The listing builds one solid part. Answer for the finished solid, in the listing's coordinates (mm). A direction names the side the tool comes from. Give positions to 0.01 mm unless a question says otherwise; leave off trailing zeros. Order: outer loops, then holes, each group sorted by start corner. A loop starts at its lowest first (then second) coordinate and runs counter-clockwise, first axis right, second up. Notation, with made-up numbers: M 18,68.25 L 39,68.25 A32 ccw 39,103.25 Z; hole C 42,-18 d2. An arc over 180 degrees is marked long. Answer as a JSON object with one key per item and string values. Group by question number.
```python
from build123d import *

# Parameters (mm, degrees)
BOSS_EXTRUDE1_DEPTH = 1.5
BOSS_EXTRUDE2_DEPTH = 3.5
CUT_EXTRUDE1_DEPTH  = 4
FILLET1_R           = 1
FILLET4_R           = 1
SKETCH5_R           = 1.5
CUT_EXTRUDE3_DEPTH  = 12
SKETCH4_R           = 1
CUT_EXTRUDE5_DEPTH  = 20


with BuildPart() as part:
    # Sketch1 → Boss-Extrude1 (new body)
    with BuildSketch(Plane.XY):
        with BuildLine():
            Line((0, 0), (20, 0))
            Line((20, 0), (20, 16))
            Line((20, 16), (18, 16))
            ThreePointArc((18, 16), (0, 22.408858912), (-18, 16))
            Line((-18, 16), (-20, 16))
            Line((-20, 16), (-20, 0))
            Line((-20, 0), (0, 0))
        make_face()
    extrude(amount=BOSS_EXTRUDE1_DEPTH)

    # Sketch2 → Boss-Extrude2 (add)
    with BuildSketch(Plane.XY.offset(1.5)):
        with BuildLine():
            Line((6, 0), (6, 13))
            ThreePointArc((6, 13), (0, 19), (-6, 13))
            Line((-6, 13), (-6, 0))
            Line((-6, 0), (6, 0))
        make_face()
    extrude(amount=BOSS_EXTRUDE2_DEPTH)

    # Sketch3 → Cut-Extrude1 (cut)
    with BuildSketch(Plane(origin=(0, 0, 0), x_dir=(-1, 0, 0), z_dir=(0, 0, -1))):
        with BuildLine():
            Line((0, 0), (5, 0))
            Line((5, 0), (5, 12))
            ThreePointArc((5, 12), (0, 17), (-5, 12))
            Line((-5, 12), (-5, 0))
            Line((-5, 0), (0, 0))
        make_face()
    extrude(amount=-CUT_EXTRUDE1_DEPTH, mode=Mode.SUBTRACT)

    # Fillet1
    fillet1_edges = [part.edges().sort_by_distance(p)[0] for p in [
        (-6, 6.5, 5),
        (0, 19, 5),
        (0, 0, 5),
        (6, 6.5, 5),
    ]]
    fillet(fillet1_edges, radius=FILLET1_R - 0.0001)  # a hair under: the kernel refuses the full size

    # Fillet4
    fillet4_edges = [part.edges().sort_by_distance(p)[0] for p in [
        (20, 8, 1.5),
        (19, 16, 1.5),
        (0, 22.408858912, 1.5),
        (13, 0, 1.5),
        (-19, 16, 1.5),
        (-20, 8, 1.5),
        (-13, 0, 1.5),
    ]]
    fillet(fillet4_edges, radius=FILLET4_R)

    # Sketch5 → Cut-Extrude3 (cut)
    with BuildSketch(Plane.XY.offset(1.5)):
        with Locations((14.499595769, 7.5)):
            Circle(SKETCH5_R)
        with Locations((-14.499595769, 7.5)):
            Circle(SKETCH5_R)
    extrude(amount=-CUT_EXTRUDE3_DEPTH, mode=Mode.SUBTRACT)

    # Sketch4 → Cut-Extrude5 (cut)
    with BuildSketch(Plane.ZY.offset(6)):
        with Locations((2.85, 7.5)):
            Circle(SKETCH4_R)
    extrude(amount=-CUT_EXTRUDE5_DEPTH, mode=Mode.SUBTRACT)


solid = part.part
```
Item 1: A tool of negligible diameter and unlimited length cuts with its end or side. For faces 4 (the cylindrical face through (18.804, 15.699, 1.215)), 5 (the flat face through (5, 6, 2)), 6 (the cylindrical face through (-18.837, 15.699, 1.215)), from which of +Z, -Z, +X, -X, +Y, -Y can it reach the whole face along a straight path? Write none if from no direction.
Item 2: Determine the mould class of faces 1 (the cylindrical face through (15.19, 6.17, 0.76)), 2 (the cylindrical face through (19.699, 8.112, 1.215)), 3 (the cylindrical face through (-12.902, 0.285, 1.199)) for opening direction Y: released by +Y, released by -Y, zero draft, split by the parting line, or undercut.
Item 3: Section A-A (y = 7.5) is taken. Count the separate pieces of the cut face and the enclosed holes in it, and give its area (3 significant figures).
Item 4: Flat-ended cylindrical pins translate along their axes: P1, Ø1.2, axis at y = 7.5, z = 2.85, coming from the +X side; P2, Ø1, axis at y = 16.5, z = 1, coming from the +X side; P3, Ø0.6, axis at x = 19, z = 0, coming from the +Y side; P4, Ø3, axis at x = -2.5, y = 8, coming from the -Z side. Find the tip coordinate at first contact, or state that the pin passes through.
Item 5: Consider probe 1 along X at (y, z) = (9, 3.35); probe 2 along Z at (x, y) = (-15, 4); probe 3 along Z at (x, y) = (3, 10.25). Determine where each line is inside the solid, lowest interval first. Write a range as from..to.
Item 6: Section B-B (z = 2.85) is taken. Determine the outline of the cut face in (x, y), and give its area (3 significant figures).
Item 7: Section C-C (y = 4.25) is taken. Determine the outline of the cut face in (x, z), and give its area (3 significant figures).
Values found:
{
 "1": {"face 4": "+Z, +X, +Y", "face 5": "-Z, -Y", "face 6": "+Z, -X, +Y"},
 "2": {"face 1": "undercut", "face 2": "zero draft", "face 3": "released by -Y"},
 "3": {"separate pieces": "5", "enclosed holes": "0", "area": "48.1 mm^2"},
 "4": {"P1": "passes through", "P2": "stops at x = 17.88", "P3": "stops at y = 16", "P4": "stops at z = 4"},
 "5": {"probe 1": "x = -6..-5, 5..6", "probe 2": "z = 0..1.5", "probe 3": "z = 4..5"},
 "6": {"outline": "M -6,0 L -5,0 L -5,6.5 L -6,6.5 Z; M -6,8.5 L -5,8.5 L -5,12 A5 cw 5,12 L 5,8.5 L 6,8.5 L 6,13 A6 ccw -6,13 Z; M 5,0 L 6,0 L 6,6.5 L 5,6.5 Z", "area": "49.3 mm^2"},
 "7": {"outline": "M -20,0 L -5,0 L -5,4 L 5,4 L 5,0 L 20,0 L 20,0.5 A1 ccw 19,1.5 L 6,1.5 L 6,4 A1 ccw 5,5 L -5,5 A1 ccw -6,4 L -6,1.5 L -19,1.5 A1 ccw -20,0.5 Z", "area": "61.1 mm^2"}
}
